Part model, mm, in its own coordinate system. Give positions to 0.01 mm unless a question says otherwise; leave off trailing zeros. Write each loop counter-clockwise with the first axis right and the second up, starting at its lowest first coordinate (ties: lowest second). Pieces come first, ordered by that corner, then holes. Notation, with made-up numbers: M -0.5,59 L 7.5,59 A15 ccw 7.5,74 Z; hole C -39,-31 d7. An arc over 180 degrees is marked long. Use a Markdown table: item, result. Add a question column.
from build123d import *

# Parameters (mm, degrees)
SKETCH_2_R = 6


with BuildPart() as part:
    # По траектории1: sweep along a path in Эскиз1
    with BuildLine(Plane(origin=(0, 0, 0), x_dir=(1, 0, 0), z_dir=(0, 1, 0))) as sweep_1_path:
        Line((18, 750), (18, 70.710678119))
        ThreePointArc((18, 70.710678119), (14.193976626, 51.5765065), (3.355339059, 35.355339059))
        Line((3.355339059, 35.355339059), (-35.355339059, -3.355339059))
        ThreePointArc((-35.355339059, -3.355339059), (-51.5765065, -14.193976626), (-70.710678119, -18))
        Line((-70.710678119, -18), (-750, -18))
    # Эскиз2 → По траектории1 (sweep)
    with BuildSketch(Plane(origin=(-750, -400, -12), x_dir=(0, 0, 1), z_dir=(-1, 0, 0))):
        with Locations((30, 400)):
            Circle(SKETCH_2_R)
    sweep(path=sweep_1_path.line)


solid = part.part
1. Cut at A-A (x = -424). Write the cut outline in (y, z), then the cut area to 3 significant figures.
2. Flat gauge pins, fed straight in: pin 1 (1.5 mm diameter, centred on x = -153, y = -3, fed in from -Z); pin 2 (1 mm diameter, centred on x = -268.5, y = 1.5, fed in from +Z); pin 3 (1.5 mm diameter, centred on x = -218, y = -4.5, fed in from -Z). Where does each tip first touch, or does it go through?
3. Drill centre lines: probe 1 along Z at (x, y) = (-102, 1); probe 2 along X at (y, z) = (-1.5, -72); probe 3 along X at (y, z) = (-0.75, -382.5). Where is each one in solid material? Low to high. Write a range as [from, to].
A:
| question | item | result |
|---|---|---|
| 1 | outline | C 0,18 d12 |
| 1 | area | 113 mm² |
| 2 | pin 1 | stops at z = 12.44 |
| 2 | pin 2 | stops at z = 23.92 |
| 2 | pin 3 | stops at z = 13.32 |
| 3 | probe 1 | z = [12.08, 23.92] |
| 3 | probe 2 | x = [12.19, 23.81] |
| 3 | probe 3 | x = [12.05, 23.95] |
